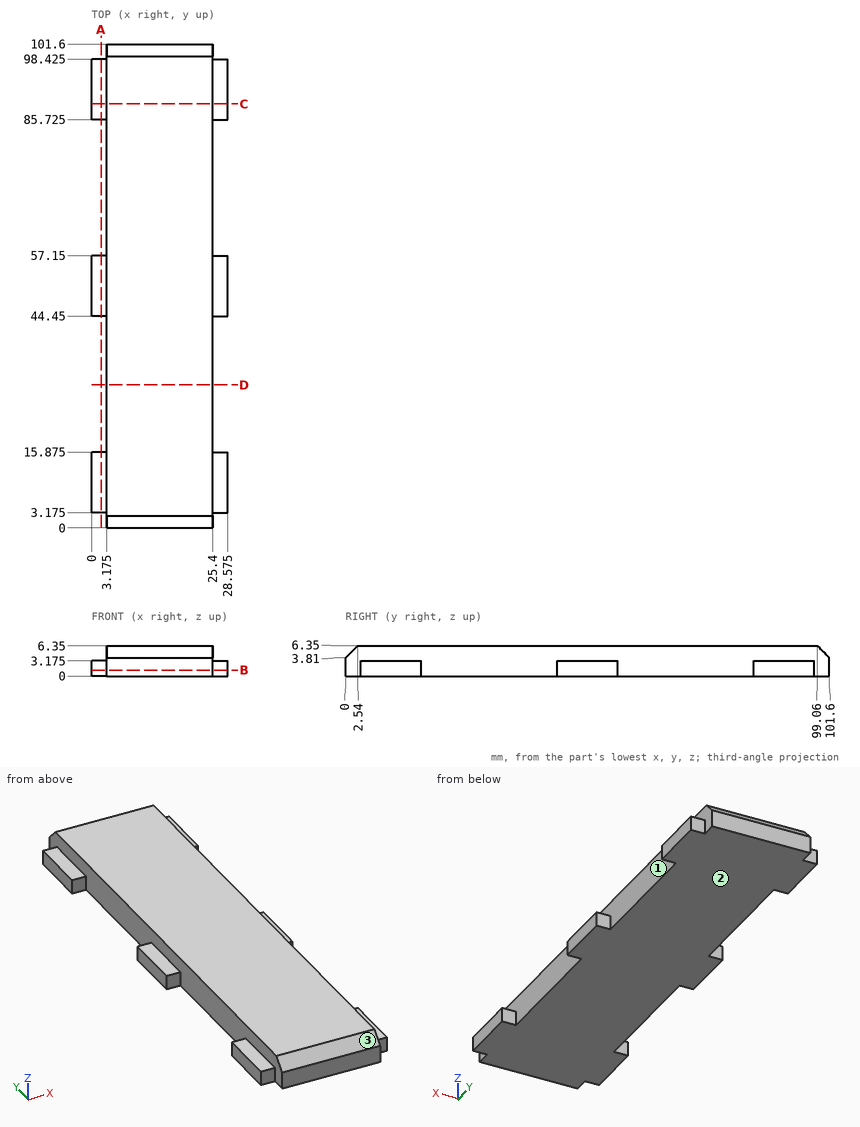
Study the drawing (mm; zero at the part's minimum x, y, z) and answer. Give positions to 0.01 mm unless a question says otherwise; leave off trailing zeros. Write each loop counter-clockwise with the first axis right and the second up, starting at its lowest first coordinate (ties: lowest second). Pieces come first, ordered by that corner, then holes. Notation, with made-up numbers: (79, 3.25) -> (103, 3.25) arc R20 cw to (103, 35.25) -> close; hole circle Ø1 at (18.25, 79). An arc over 180 degrees is marked (long way). Write item = value, one per line. Start each with the question number.
1) The part is cut by section B-B, the plane z = 1.25. Determine the outline of the cut face in (x, y) (3 decimals).
2) Each of these flat-tipped pins is pushed along its axis until it touches: pin 1 (1 mm diameter, centred on x = 2, z = 1.5, fed in from +Y) (3 decimals); pin 2 (1 mm diameter, centred on x = 2, y = 89.5, fed in from +Z) (3 decimals); pin 3 (2.5 mm diameter, centred on x = 27.5, z = 2, fed in from -Y) (3 decimals). Where does it stop, or does it pass through?
3) Determine the mould class of the marked faces 1, 2 and 3 for opening direction Y: +Y half, -Y half, draft (parallel to the pull), parting line (faces both ways), or undercut.
4) The part is cut by section D-D, the plane y = 30. Determine the outline of the cut face in (x, z) (3 decimals).
5) The part is cut by section A-A, the plane x = 2. Determine the outline of the cut face in (y, z) (3 decimals).
6) Straight lines are drawn through the part: line 1 along X through (y, z) = (16, 1) (3 decimals); line 2 along Y through (x, z) = (15.5, 4); line 3 along Y through (x, z) = (15.5, 6). For each, find the intervals that lie inside material, in ascending order.
7) The part is cut by section C-C, the plane y = 89. Determine the outline of the cut face in (x, z) (3 decimals).
Solutions:
q1.outline = (0, 3.175) -> (3.175, 3.175) -> (3.175, 0) -> (25.4, 0) -> (25.4, 3.175) -> (28.575, 3.175) -> (28.575, 15.875) -> (25.4, 15.875) -> (25.4, 44.45) -> (28.575, 44.45) -> (28.575, 57.15) -> (25.4, 57.15) -> (25.4, 85.725) -> (28.575, 85.725) -> (28.575, 98.425) -> (25.4, 98.425) -> (25.4, 101.6) -> (3.175, 101.6) -> (3.175, 98.425) -> (0, 98.425) -> (0, 85.725) -> (3.175, 85.725) -> (3.175, 57.15) -> (0, 57.15) -> (0, 44.45) -> (3.175, 44.45) -> (3.175, 15.875) -> (0, 15.875) -> close
q2.pin_1 = 98.425
q2.pin_2 = 3.175
q2.pin_3 = 3.175
q3.face_1 = undercut
q3.face_2 = draft
q3.face_3 = -Y half
q4.outline = (3.175, 0) -> (25.4, 0) -> (25.4, 6.35) -> (3.175, 6.35) -> close
q5.outline = (3.175, 0) -> (15.875, 0) -> (15.875, 3.175) -> (3.175, 3.175) -> close; (44.45, 0) -> (57.15, 0) -> (57.15, 3.175) -> (44.45, 3.175) -> close; (85.725, 0) -> (98.425, 0) -> (98.425, 3.175) -> (85.725, 3.175) -> close
q6.line_1 = 3.175 to 25.4
q6.line_2 = 0.19 to 101.41
q6.line_3 = 2.19 to 99.41
q7.outline = (0, 0) -> (28.575, 0) -> (28.575, 3.175) -> (25.4, 3.175) -> (25.4, 6.35) -> (3.175, 6.35) -> (3.175, 3.175) -> (0, 3.175) -> close
